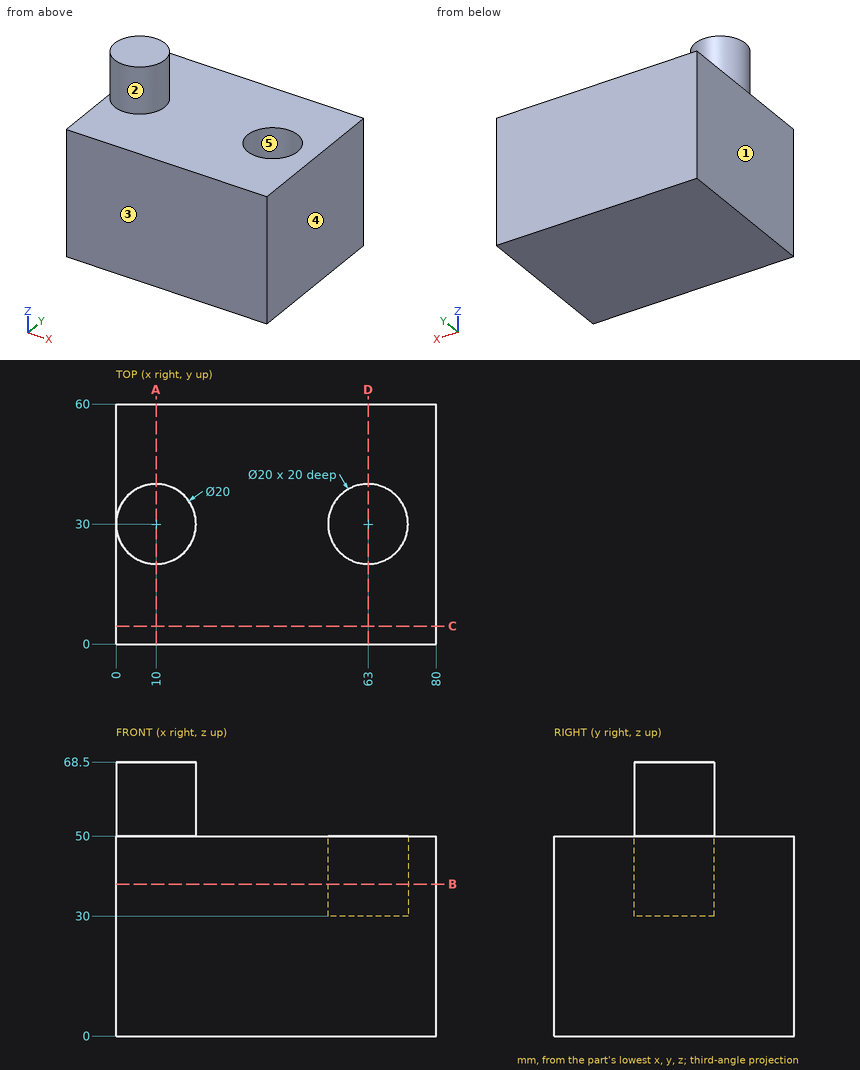
Study the drawing (mm; zero at the part's minimum x, y, z) and answer. A direction names the side the tool comes from. Coordinates: 2 decimals unless noted, no trailing zeros. Write each loop counter-clockwise with the first axis right and the second up, starting at its lowest first coordinate (ties: lowest second). Pieces come first, ordered by that corner, then holes. Notation, with made-up numbers: (64.25, 74.5) - (107.25, 74.5) arc R27 ccw to (107.25, 110.5) - close; hole circle Ø1 at (57.25, -29). An arc over 180 degrees is marked (long way). One line per item, written item: value.
1) Find section B-B (z = 38). Give the vertices of the cut face in (x, y), and give its area (3 significant figures).
Geometry check:
outline: (0, 0) - (80, 0) - (80, 60) - (0, 60) - close; hole circle Ø20 at (63, 30)
area: 4,490 mm2
2) Find section A-A (x = 10). Give the vertices of the cut face in (y, z), and give its area (3 significant figures).
Geometry check:
outline: (0, 0) - (60, 0) - (60, 50) - (40, 50) - (40, 68.5) - (20, 68.5) - (20, 50) - (0, 50) - close
area: 3,370 mm2
3) A tool of negligible diameter and unlimited length cuts with its end or side. For the marked faces 1 and 2, from which of +Z, -Z, +X, -X, +Y, -Y can it reach the whole face along a straight path? Write none if from no direction.
Geometry check:
face 1: +Z, -Z, -X, +Y, -Y
face 2: +Z
4) Find section C-C (y = 4.5). Give the vertices of the cut face in (x, z), and give its area (3 significant figures).
Geometry check:
outline: (0, 0) - (80, 0) - (80, 50) - (0, 50) - close
area: 4,000 mm2
5) For a pull along Y with two mould halves and no side action, classify the marked faces 3, 4 and 5 as pulls with the +Y half, pulls with the -Y half, needs draft (parallel to the pull), parting line crosses it, or undercut.
Geometry check:
face 3: pulls with the -Y half
face 4: needs draft
face 5: undercut
6) Consider line 1 along Y through (x, z) = (63, 42); line 2 along Z through (x, y) = (67, 51.5); line 3 along Y through (x, z) = (67, 36.5). Determine where each line is inside the solid, lowest interval first. Write a range as from..to.
Geometry check:
line 1: y = 0..20, 40..60
line 2: z = 0..50
line 3: y = 0..20.83, 39.17..60
7) Each of these flat-tipped pins is pushed along its axis until it touches: pin 1 Ø6 at (x, y) = (59, 30) entering from +Z; pin 2 Ø1.5 at (y, z) = (39.5, 55) entering from +X. Where does it stop, or does it pass through?
Geometry check:
pin 1: stops at z = 30
pin 2: stops at x = 14.84
8) Find section D-D (x = 63). Give the vertices of the cut face in (y, z).
Geometry check:
outline: (0, 0) - (60, 0) - (60, 50) - (40, 50) - (40, 30) - (20, 30) - (20, 50) - (0, 50) - close
